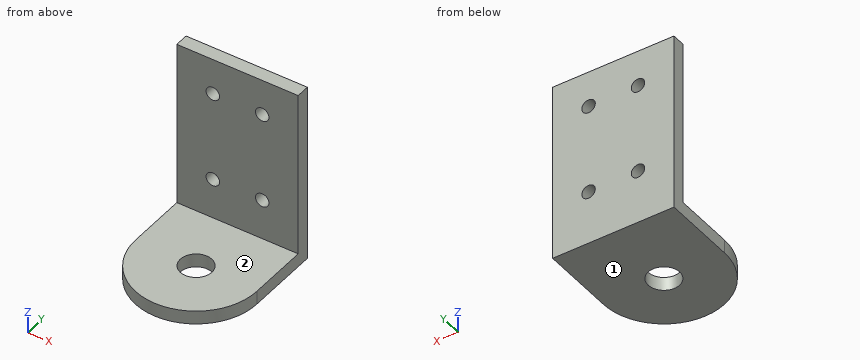
from build123d import *

# Parameters (mm, degrees)
MODEL_R             = 3.5
EXTRUDE_1_DEPTH     = 40
SKETCH_3_W          = 37
SKETCH_3_H          = 37
CUT_EXTRUDE_1_DEPTH = 40
SKETCH_4_R          = 1.5
CUT_EXTRUDE_2_DEPTH = 40


with BuildPart() as part:
    # Model → 凸台-拉伸1 (new body)
    with BuildSketch(Plane.XY):
        with BuildLine():
            Line((2619.766714505, 1592.826425633), (2619.766714505, 1609.326425633))
            Line((2619.766714505, 1609.326425633), (2592.766714505, 1609.326425633))
            Line((2592.766714505, 1609.326425633), (2592.766714505, 1592.826425633))
            ThreePointArc((2592.766714505, 1592.826425633), (2606.266714505, 1579.326425633), (2619.766714505, 1592.826425633))
        make_face()
        with Locations((2606.266714505, 1592.826425633)):
            Circle(MODEL_R, mode=Mode.SUBTRACT)
    extrude(amount=EXTRUDE_1_DEPTH)

    # 草图3 → 切除-拉伸1 (cut)
    with BuildSketch(Plane(origin=(2619.766714505, 0, 0), x_dir=(0, 0, -1), z_dir=(1, 0, 0))):
        with Locations((-21.5, 1587.826425633)):
            Rectangle(SKETCH_3_W, SKETCH_3_H)
    extrude(amount=-CUT_EXTRUDE_1_DEPTH, mode=Mode.SUBTRACT)

    # 草图4 → 切除-拉伸2 (cut)
    with BuildSketch(Plane(origin=(0, 1609.326425633, 0), x_dir=(1, 0, 0), z_dir=(0, 1, 0))):
        with Locations((2600.766714505, -32)):
            Circle(SKETCH_4_R)
        with Locations((2611.766714505, -32)):
            Circle(SKETCH_4_R)
        with Locations((2600.766714505, -12)):
            Circle(SKETCH_4_R)
        with Locations((2611.766714505, -12)):
            Circle(SKETCH_4_R)
    extrude(amount=-CUT_EXTRUDE_2_DEPTH, mode=Mode.SUBTRACT)


solid = part.part
Source: CAD feature listing. Evaluate the final solid. Frame: model axes, mm. Face numbers are marked on the shaded views. A direction names the side the tool comes from. Give positions to 0.01 mm unless a question says otherwise; leave off trailing zeros. Write each loop counter-clockwise with the first axis right and the second up, starting at its lowest first coordinate (ties: lowest second). Pieces come first, ordered by that corner, then holes. Notation, with made-up numbers: (-16.75, 16.25) -> (3.25, 16.25) arc R20 ccw to (3.25, 28.25) -> close; hole circle Ø1 at (3.25, 10). An arc over 180 degrees is marked (long way). Return JSON: item names as keys, results as strings. Group by question number.
1. Section B-B, the plane y = 1594.5. Output: boundary loops of the cut face in (x, z).
2. Section D-D, the plane y = 1604.25. Output: boundary loops of the cut face in (x, z), then the cut area to 3 significant figures.
3. Material intervals for line 1 (X direction, y = 1608.2, z = 12); line 2 (Y direction, x = 2607, z = 33); line 3 (Z direction, x = 2610.75, y = 1586.25), sorted ascending. Write a range as from..to.
4. Access query for the marked faces 1 and 2. Directions: +Z, -Z, +X, -X, +Y, -Y. A direction counts if a zero-diameter tool reaches every point of the face in a straight line with its end or side. Return the directions, or none.
5. Pin query (flat end, axial travel): pin 1 Ø1.5 at (x, z) = (2598.5, 28.5) entering from -Y; pin 2 Ø8 at (x, y) = (2604.5, 1602.5) entering from -Z; pin 3 Ø13.5 at (x, y) = (2605, 1597) entering from +Z. Return the tip coordinate at first contact, or that it passes through.
6. Section A-A, the plane z = 12. Output: boundary loops of the cut face in (x, y).
7. Section C-C, the plane x = 2606. Output: boundary loops of the cut face in (y, z), then the cut area to 3 significant figures.
Determined:
{
 "1": {"outline": "(2592.77, 0) -> (2603.19, 0) -> (2603.19, 3) -> (2592.77, 3) -> close; (2609.34, 0) -> (2619.77, 0) -> (2619.77, 3) -> (2609.34, 3) -> close"},
 "2": {"outline": "(2592.77, 0) -> (2619.77, 0) -> (2619.77, 3) -> (2592.77, 3) -> close", "area": "81.0 mm2"},
 "3": {"line 1": "x = 2592.77..2599.27, 2602.27..2610.27, 2613.27..2619.77", "line 2": "y = 1606.33..1609.33", "line 3": "z = 0..3"},
 "4": {"face 1": "-Z, +X, -X, +Y, -Y", "face 2": "+Z, +X, -X, -Y"},
 "5": {"pin 1": "stops at y = 1606.33", "pin 2": "stops at z = 0", "pin 3": "stops at z = 3"},
 "6": {"outline": "(2592.77, 1606.33) -> (2599.27, 1606.33) -> (2599.27, 1609.33) -> (2592.77, 1609.33) -> close; (2602.27, 1606.33) -> (2610.27, 1606.33) -> (2610.27, 1609.33) -> (2602.27, 1609.33) -> close; (2613.27, 1606.33) -> (2619.77, 1606.33) -> (2619.77, 1609.33) -> (2613.27, 1609.33) -> close"},
 "7": {"outline": "(1579.33, 0) -> (1589.34, 0) -> (1589.34, 3) -> (1579.33, 3) -> close; (1596.32, 0) -> (1609.33, 0) -> (1609.33, 40) -> (1606.33, 40) -> (1606.33, 3) -> (1596.32, 3) -> close", "area": "180 mm2"}
}
